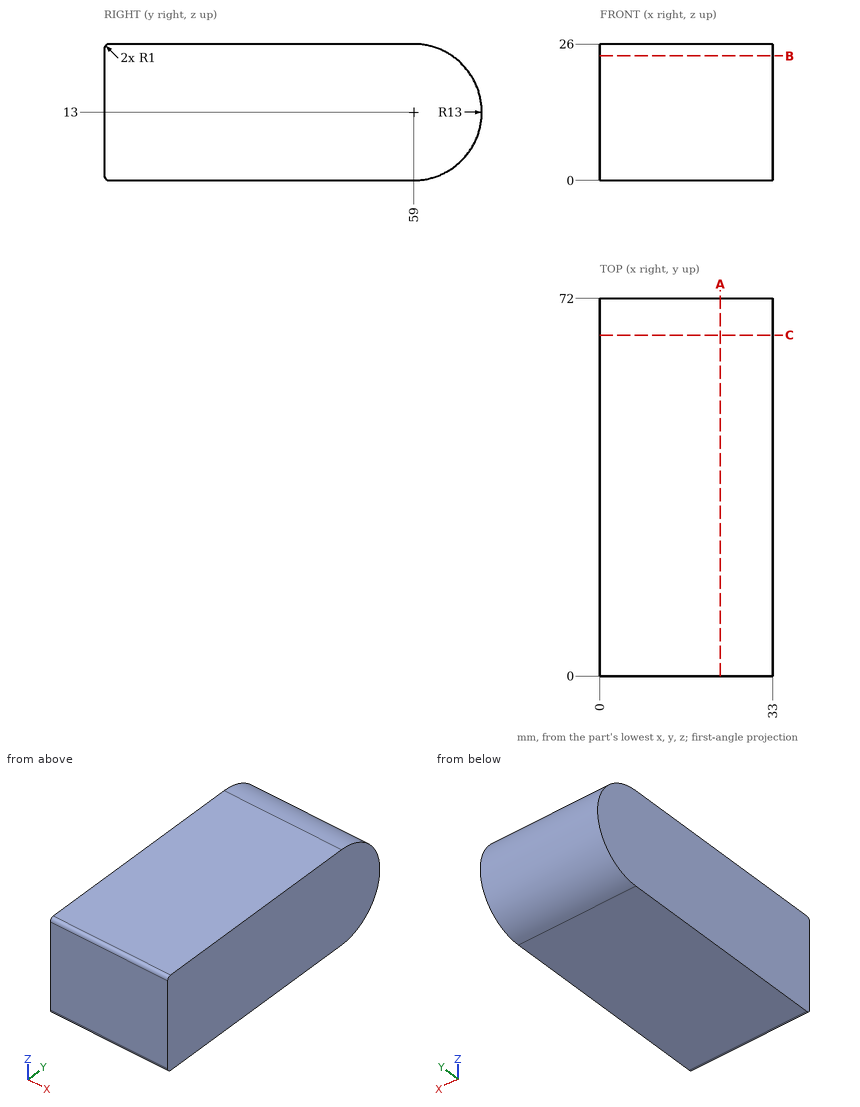
Print and shaded views of the part. All mm, measured from the part's lowest x, y and z. Coordinates: 2 decimals unless noted, no trailing zeros. Loops run counter-clockwise (first coordinate to the right, second up) from the corner with the lowest first, then second, coordinate; pieces in that order, holes last. Notation, with made-up numbers: (39, 59) - (82, 59) arc R17 ccw to (82, 79) - close; hole circle Ø4 at (81.25, -26.75). An arc over 180 degrees is marked (long way). Write item = value, one per line. Start each with the question number.
Item 1: Wall check: L1, parallel to Y at x = 27, z = 12.5; L2, parallel to Z at x = 26, y = 68; L3, parallel to Y at x = 5.5, z = 4.5. Give the ranges that are in metal, low to high. Write a range as from..to.
Item 2: Cut at A-A, the plane x = 23. Give the cut face in (y, z).
Item 3: Cut at B-B, the plane z = 23.75. Give the cut face in (x, y).
Item 4: Cut at C-C, the plane y = 65. Give the cut face in (x, z), and give its area (3 significant figures).
The answers:
q1.L1 = 0..71.99
q1.L2 = 3.62..22.38
q1.L3 = 0..68.84
q2.outline = (0, 1) arc R1 ccw to (1, 0) - (59, 0) arc R13 ccw to (59, 26) - (1, 26) arc R1 ccw to (0, 25) - close
q3.outline = (0, 0) - (33, 0) - (33, 66.31) - (0, 66.31) - close
q4.outline = (0, 1.47) - (33, 1.47) - (33, 24.53) - (0, 24.53) - close
q4.area = 761 mm2
